Source: CAD feature listing. Evaluate the final solid. Frame: model axes, mm. Face numbers are marked on the shaded views. A direction names the side the tool comes from. Give positions to 0.01 mm unless a question says otherwise; leave off trailing zeros. Order: outer loops, then holes, each group sorted by start corner. A loop starts at its lowest first (then second) coordinate and runs counter-clockwise, first axis right, second up.
from build123d import *

# Parameters (mm, degrees)
EXTRUDE_1_DEPTH     = 80
SKETCH_2_R          = 7.5
CUT_EXTRUDE_1_DEPTH = 3
SKETCH_3_R          = 4.25
CUT_EXTRUDE_2_DEPTH = 3
SKETCH_4_R          = 5
CUT_EXTRUDE_3_DEPTH = 20


with BuildPart() as part:
    # Sketch 1 → Extrude 1 (new body)
    with BuildSketch(Plane.XY):
        with BuildLine():
            Line((8.5, -12.5), (-8.5, -12.5))
            ThreePointArc((-8.5, -12.5), (-11.328427125, -11.328427125), (-12.5, -8.5))
            Line((-12.5, -8.5), (-12.5, 8.5))
            ThreePointArc((-12.5, 8.5), (-11.328427125, 11.328427125), (-8.5, 12.5))
            Line((-8.5, 12.5), (8.5, 12.5))
            ThreePointArc((8.5, 12.5), (11.328427125, 11.328427125), (12.5, 8.5))
            Line((12.5, 8.5), (12.5, -8.5))
            ThreePointArc((12.5, -8.5), (11.328427125, -11.328427125), (8.5, -12.5))
        make_face()
        with BuildLine():
            Line((-10.5, -8.5), (-10.5, 8.5))
            ThreePointArc((-10.5, 8.5), (-9.914213562, 9.914213562), (-8.5, 10.5))
            Line((-8.5, 10.5), (8.5, 10.5))
            ThreePointArc((8.5, 10.5), (9.914213562, 9.914213562), (10.5, 8.5))
            Line((10.5, 8.5), (10.5, -8.5))
            ThreePointArc((10.5, -8.5), (9.914213562, -9.914213562), (8.5, -10.5))
            Line((8.5, -10.5), (-8.5, -10.5))
            ThreePointArc((-8.5, -10.5), (-9.914213562, -9.914213562), (-10.5, -8.5))
        make_face(mode=Mode.SUBTRACT)
    extrude(amount=EXTRUDE_1_DEPTH)

    # Sketch 2 → Cut-Extrude 1 (cut)
    with BuildSketch(Plane(origin=(12.5, 0, 0), x_dir=(0, 0, -1), z_dir=(1, 0, 0))):
        with Locations((-40, 0)):
            Circle(SKETCH_2_R)
    extrude(amount=-CUT_EXTRUDE_1_DEPTH, mode=Mode.SUBTRACT)

    # Sketch 3 → Cut-Extrude 2 (cut)
    with BuildSketch(Plane.ZY.offset(12.5)):
        with Locations((40, 0)):
            Circle(SKETCH_3_R)
    extrude(amount=-CUT_EXTRUDE_2_DEPTH, mode=Mode.SUBTRACT)

    # Sketch 4 → Cut-Extrude 3 (cut)
    with BuildSketch(Plane(origin=(0, 0, 0), x_dir=(0, 0, -1), z_dir=(0.7071067811865488, 0.7071067811865464, 0))):
        with Locations(Location((-15, 0, 0), (0, 0, 214.449901988))):
            Circle(SKETCH_4_R)
    extrude(amount=CUT_EXTRUDE_3_DEPTH, mode=Mode.SUBTRACT)


solid = part.part
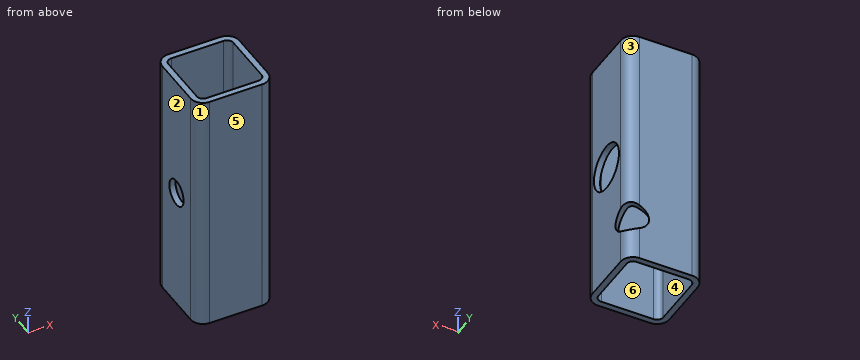
1) Section query C-C on y = 0. Output: boundary loops of the cut face in (x, z).
Checks:
outline: (-12.5, 0) - (-10.5, 0) - (-10.5, 35.75) - (-12.5, 35.75) - close; (-12.5, 44.25) - (-10.5, 44.25) - (-10.5, 80) - (-12.5, 80) - close; (10.5, 0) - (12.5, 0) - (12.5, 32.5) - (10.5, 32.5) - close; (10.5, 47.5) - (12.5, 47.5) - (12.5, 80) - (10.5, 80) - close
2) Pull-direction query (Y, two-part tool) for the marked faces 1, 2, 3 and 4; classes: +Y half, -Y half, draft (parallel to the pull), parting line (faces both ways), or undercut.
Checks:
face 1: -Y half
face 2: draft
face 3: +Y half
face 4: undercut
3) Ray query, L1, parallel to X at y = -7, z = 66.5; L2, parallel to X at y = 0, z = 47. Return the intervals inside material, ascending.
Checks:
L1: x = -12.5 to -10.5, 10.5 to 12.5
L2: x = -12.5 to -10.5
4) Section query A-A on x = -5.25. Output: boundary loops of the cut face in (y, z), and give its area (3 significant figures).
Checks:
outline: (-12.5, 0) - (-10.5, 0) - (-10.5, 80) - (-12.5, 80) - close; (10.5, 0) - (12.5, 0) - (12.5, 80) - (10.5, 80) - close
area: 320 mm2
5) First-contact query: pin 1 Ø12 at (y, z) = (0, 40) entering from +X; pin 2 Ø5 at (y, z) = (0, 40) entering from +X. Flat tips, straight axial feed; report the tip coordinate or a pass-through.
Checks:
pin 1: stops at x = -10.5
pin 2: passes through
6) Section query D-D on z = 70. Output: boundary loops of the cut face in (x, y), and give its area (3 significant figures).
Checks:
outline: (-12.5, -8.5) arc R4 ccw to (-8.5, -12.5) - (8.5, -12.5) arc R4 ccw to (12.5, -8.5) - (12.5, 8.5) arc R4 ccw to (8.5, 12.5) - (-8.5, 12.5) arc R4 ccw to (-12.5, 8.5) - close; hole (-10.5, -8.5) arc R2 ccw to (-8.5, -10.5) - (8.5, -10.5) arc R2 ccw to (10.5, -8.5) - (10.5, 8.5) arc R2 ccw to (8.5, 10.5) - (-8.5, 10.5) arc R2 ccw to (-10.5, 8.5) - close
area: 174 mm2
7) Reachability of the marked faces 5 and 6 from +Z, -Z, +X, -X, +Y, -Y: full face, straight path, thin tool, end or side. Return the list, or none.
Checks:
face 5: +Z, -Z, +X, -X, -Y
face 6: +Z, -Z
8) Section query B-B on z = 40. Output: boundary loops of the cut face in (x, y).
Checks:
outline: (-12.5, -8.5) arc R4 ccw to (-8.5, -12.5) - (8.5, -12.5) arc R4 ccw to (12.5, -8.5) - (12.5, -7.5) - (10.5, -7.5) - (10.5, -8.5) arc R2 cw to (8.5, -10.5) - (-8.5, -10.5) arc R2 cw to (-10.5, -8.5) - (-10.5, -4.25) - (-12.5, -4.25) - close; (-12.5, 4.25) - (-10.5, 4.25) - (-10.5, 8.5) arc R2 cw to (-8.5, 10.5) - (8.5, 10.5) arc R2 cw to (10.5, 8.5) - (10.5, 7.5) - (12.5, 7.5) - (12.5, 8.5) arc R4 ccw to (8.5, 12.5) - (-8.5, 12.5) arc R4 ccw to (-12.5, 8.5) - close
